```python
from build123d import *

# Parameters (mm, degrees)
F0_W     = 200
F0_H     = 50.8
F1_DEPTH = 83
F3_DEPTH = 83
F4_DEPTH = 83
F5_T     = -3
F7_DEPTH = 101.6


with BuildPart() as f1:
    # F0 (on Right) → F1 (new body)
    with BuildSketch(Plane.YZ):
        Rectangle(F0_W, F0_H)
    extrude(amount=F1_DEPTH)

    # F2 (on face) → F3 (cut)
    with BuildSketch(Plane.YZ.offset(83)):
        Polygon((-100, -8.856749), (0, 25.4), (-100, 25.4), align=None)
    extrude(amount=-F3_DEPTH, mode=Mode.SUBTRACT)

    # F2 (on face) → F4 (join)
    with BuildSketch(Plane.YZ.offset(83)):
        Polygon((0, -25.4), (0, 25.4), (-148.291945, -25.4), align=None)
    extrude(amount=-F4_DEPTH)

    # F5
    f5_openings = [f1.faces().sort_by_distance(p)[0] for p in [
        (41.5, -24.145973, -25.4),
    ]]
    offset(amount=F5_T, openings=f5_openings)

    # F6 (on face) → F7 (cut)
    with BuildSketch(Plane.YZ.offset(83)):
        with BuildLine():
            Line((-76.226585, -25.4), (-46.226585, -25.4))
            ThreePointArc((-46.226585, -25.4), (-61.226585, -10.4), (-76.226585, -25.4))
        make_face()
        with BuildLine():
            ThreePointArc((69.692981, -25.4), (54.694057, -10.220377), (39.695133, -25.4))
            Line((39.695133, -25.4), (69.692981, -25.4))
        make_face()
    extrude(amount=-F7_DEPTH, mode=Mode.SUBTRACT)


solid = f1.part
```
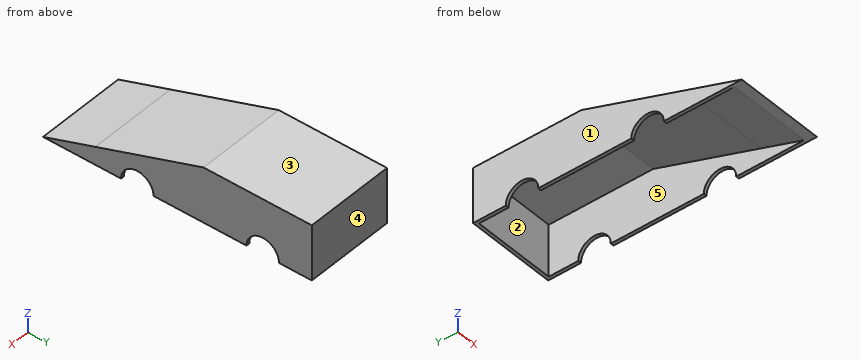
Check sheet for the modelled part. Datum: model origin and axes. Units: mm. Face numbers are marked on the shaded views. A direction names the side the tool comes from. Round coordinates to 2 decimals unless told otherwise and drop trailing zeros. Order: outer loops, then holes, each group sorted by start corner. A loop starts at its lowest first (then second) coordinate and runs counter-clockwise, first axis right, second up. Notation, with made-up numbers: (49.5, -27.75) - (72.5, -27.75) arc R26 ccw to (72.5, 0.25) - close; hole circle Ø10 at (55.5, 9.25). An arc over 180 degrees is marked (long way). Answer as CSV lines item,"result". Start each with the question number.
1) Section check B-B (z = -1.5). Record the cut outline in (x, y), then the cut area to 3 significant figures.
2) Section check A-A (x = 13). Record the cut outline in (y, z), then the cut area to 3 significant figures.
3) Tool access check on the marked faces 1 and 2. Record the directions out of +Z, -Z, +X, -X, +Y, -Y that give a thin tool (end or side, any length) a straight path to the whole face; none if there is none.
4) Section check D-D (y = -86). Record the cut outline in (x, z), then the cut area to 3 significant figures.
5) Depth check by flat-ended pin: pin 1 (1 mm diameter, centred on x = 26.5, y = -121, fed in from -Z); pin 2 (1 mm diameter, centred on x = 37, y = -66.5, fed in from -Z); pin 3 (14.5 mm diameter, centred on y = -70.5, z = 8.5, fed in from +X); pin 4 (3 mm diameter, centred on x = 37.5, y = -28, fed in from +Z). Enter the tip coordinate at first touch or a pass-through.
6) Draft check along Y on the marked faces 3, 4 and 5. Enter one of: +Y half, -Y half, draft (parallel to the pull), parting line (faces both ways), or undercut.
7) Section check C-C (z = -21.5). Record the cut outline in (x, y).
8) Scan lines: probe 1 along X at (y, z) = (28.5, 16); probe 2 along Z at (x, y) = (24, 42); probe 3 along Z at (x, y) = (31, -83.5). Record each from-to range of solid material in increasing order.
Determined:
1,outline,"(0, -78.52) - (83, -78.52) - (83, 100) - (0, 100) - close; hole (3, -69.27) - (80, -69.27) - (80, 97) - (3, 97) - close"
1,area,"2,010 mm^2"
2,outline,"(-148.29, -25.4) - (-139.03, -25.4) - (0.5, 22.4) - (97, 22.4) - (97, -25.4) - (100, -25.4) - (100, 25.4) - (0, 25.4) - close"
2,area,"899 mm^2"
3,face 1,"+Z, -Z, -X, +Y, -Y"
3,face 2,"-Z"
4,outline,"(0, -25.4) - (3, -25.4) - (3, -7.23) - (80, -7.23) - (80, -25.4) - (83, -25.4) - (83, -4.06) - (0, -4.06) - close"
4,area,"372 mm^2"
5,pin 1,"z = -19.39"
5,pin 2,"z = -0.72"
5,pin 3,"x = 83"
5,pin 4,"z = 16.32"
6,face 3,"draft"
6,face 4,"+Y half"
6,face 5,"undercut"
7,outline,"(0, -136.91) - (83, -136.91) - (83, -75.71) - (80, -75.71) - (80, -127.65) - (3, -127.65) - (3, -75.71) - (0, -75.71) - close; (0, -46.74) - (3, -46.74) - (3, 40.16) - (0, 40.16) - close; (0, 69.23) - (3, 69.23) - (3, 97) - (80, 97) - (80, 69.23) - (83, 69.23) - (83, 100) - (0, 100) - close; (80, -46.74) - (83, -46.74) - (83, 40.16) - (80, 40.16) - close"
8,probe 1,"0 to 3, 80 to 83"
8,probe 2,"22.4 to 25.4"
8,probe 3,"-6.38 to -3.2"
